Answer from the drawing. Dimensions are ordinates in mm from the lowest x, y and z of the part. A direction names the side the tool comes from. Coordinates: 2 decimals unless noted, no trailing zeros. Order: outer loops, then holes, each group sorted by start corner. A loop starts at its lowest first (then second) coordinate and runs counter-clockwise, first axis right, second up. Notation, with made-up numbers: (15, 7) -> (46, 7) arc R30 ccw to (46, 35) -> close; hole circle Ø11 at (34.25, 57). An arc over 180 degrees is marked (long way). Answer as a JSON object with one key per item and string values. Group by question number.
1) Consider L1, parallel to X at y = 7, z = 6; L2, parallel to X at y = 9, z = 4.5; L3, parallel to Y at x = 33.5, z = 4. Determine where each line is inside the solid, lowest interval first.
2) Section B-B on x = 133 is taken. Determine the outline of the cut face in (y, z).
3) Section A-A on z = 5.5 is taken. Determine the outline of the cut face in (x, y).
4) Section C-C on y = 48 is taken. Determine the outline of the cut face in (x, z).
5) Given pin 1 (2.5 mm diameter, centred on y = 16.5, z = 5, fed in from -X); pin 2 (4 mm diameter, centred on x = 92.5, z = 6, fed in from -Y); pin 3 (2.5 mm diameter, centred on y = 2.5, z = 3.5, fed in from +X), each flat-ended and moving along its own axis, determine where each tip first touches the part or whether it passes through.
6) Determine the mould class of the marked faces 1, 2 and 3 for opening direction X: released by +X, released by -X, zero draft, split by the parting line, or undercut.
7) A tool of negligible diameter and unlimited length cuts with its end or side. For the marked faces 4, 5, 6, 7 and 8, from which of +Z, -Z, +X, -X, +Y, -Y can it reach the whole face along a straight path? Write none if from no direction.
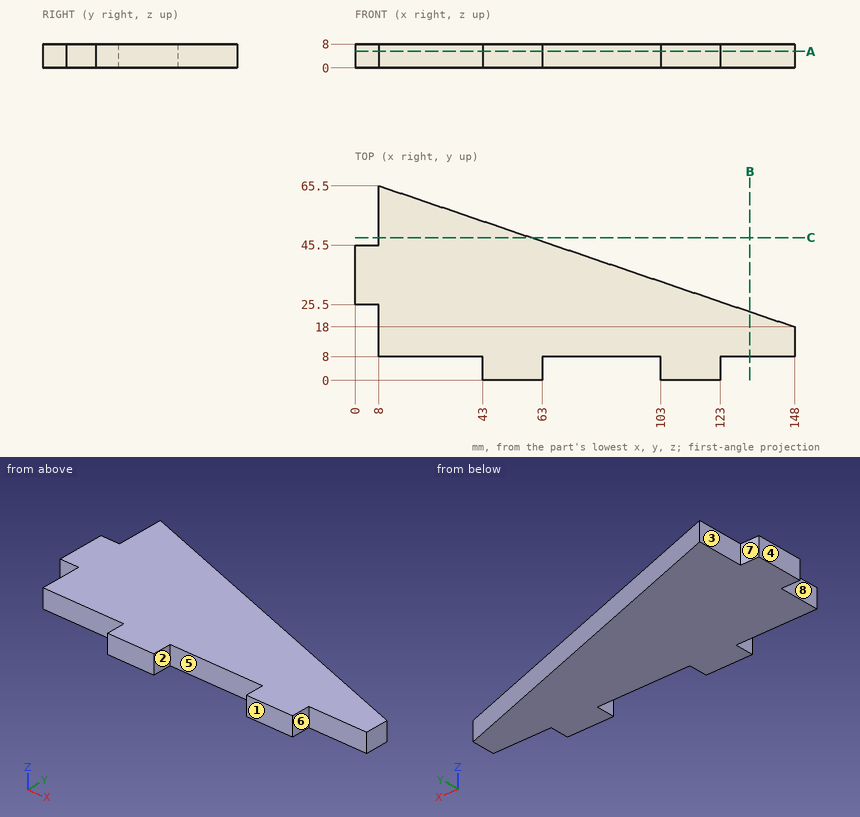
Worked answers:
{
 "1": {"L1": "x = 43 to 63, 103 to 123", "L2": "x = 8 to 148", "L3": "y = 8 to 56.85"},
 "2": {"outline": "(8, 0) -> (23.09, 0) -> (23.09, 8) -> (8, 8) -> close"},
 "3": {"outline": "(0, 25.5) -> (8, 25.5) -> (8, 8) -> (43, 8) -> (43, 0) -> (63, 0) -> (63, 8) -> (103, 8) -> (103, 0) -> (123, 0) -> (123, 8) -> (148, 8) -> (148, 18) -> (8, 65.5) -> (8, 45.5) -> (0, 45.5) -> close"},
 "4": {"outline": "(8, 0) -> (59.58, 0) -> (59.58, 8) -> (8, 8) -> close"},
 "5": {"pin 1": "stops at x = 8", "pin 2": "stops at y = 8", "pin 3": "stops at x = 123"},
 "6": {"face 1": "zero draft", "face 2": "undercut", "face 3": "released by -X"},
 "7": {"face 4": "+Z, -Z, -X, +Y, -Y", "face 5": "+Z, -Z, -Y", "face 6": "+Z, -Z, +X, -Y", "face 7": "+Z, -Z, -X, +Y", "face 8": "+Z, -Z, -X, -Y"}
}
